Autodesk Inventor part; units mm, degrees
ref_plane "YZ Plane" through (0, 0, 0) normal (1, 0, 0) x (0, 1, 0)
ref_plane "XZ Plane" through (0, 0, 0) normal (0, 1, 0) x (-1, 0, 0)
ref_plane "XY Plane" through (0, 0, 0) normal (0, 0, 1) x (1, 0, 0)
sketch "スケッチ1" plane through (0, 0, 0) normal (0, 0, 1) x (1, 0, 0)
  line L0 (-10, 30) -> (10, 30)
  line L1 (10, 30) -> (10, -30)
  line L2 (10, -30) -> (-10, -30)
  line L3 (-10, -30) -> (-10, 30)
  line L4 (-10, 30) -> (10, -30) construction
  line L5 (10, 30) -> (-10, -30) construction
  line L6 (10, 30) -> (20, 30)
  line L7 (20, 30) -> (20, 11)
  line L8 (20, 11) -> (10, 11)
  line L9 (10.5, 30) -> (10.5, 11) construction
  circle A0 centre (10.5, 24) radius 1.25
  circle A1 centre (10.5, 16) radius 1.25
  line L10 (3.5, 30) -> (3.5, 11)
  line L11 (3.5, 11) -> (-10, 11)
  circle A2 centre (-6.25, -26.44) radius 1.1
  line L12 (-10, -26.44) -> (10, -26.44) construction
  circle A3 centre (6.25, -26.44) radius 1.1
  line L13 (0, -30) -> (0, 30) construction
  line L14 (-9.5, -15.94) -> (9.5, -15.94)
  line L15 (9.5, -15.94) -> (9.5, -18.94)
  line L16 (9.5, -18.94) -> (-9.5, -18.94)
  line L17 (-9.5, -18.94) -> (-9.5, -15.94)
  line L18 (-9.5, -15.94) -> (9.5, -18.94) construction
  line L19 (9.5, -15.94) -> (-9.5, -18.94) construction
  line L20 (10, 11) -> (3.5, 11)
  circle A4 centre (6.25, -26.44) radius 2.5
  circle A5 centre (-6.25, -26.44) radius 2.5
  line L21 (10, -30) -> (12, -30)
  line L22 (12, -30) -> (12, 11)
  line L23 (-10, 11) -> (-12, 11)
  line L24 (-12, 11) -> (-12, -30)
  line L25 (-12, -30) -> (-10, -30)
  point P0 (0, 0)
  point P1 (0, -17.44)
  dimension "d0" = 60
  dimension "d1" = 20
  dimension "d2" = 2.5
  dimension "d3" = 8
  dimension "d4" = 5
  dimension "d5" = 10.5
  dimension "d6" = 19
  dimension "d7" = 10
  dimension "d8" = 7
  dimension "d9" = 2.2
  dimension "d10" = 2.2
  dimension "d11" = 12.5
  dimension "d12" = 6.25
  dimension "d13" = 3.56
  dimension "d14" = 3
  dimension "d15" = 19
  dimension "d16" = 9
  dimension "d22" = 5
  dimension "d23" = 5
  dimension "d27" = 2
  dimension "d28" = 2
extrude "押し出し1" add sketch "スケッチ1" along normal blind 2 contours L0 L1 A0 A1 L20 L10 | L11 L20 L1 L2 L3 | L6 L7 L8 L1 A1 A0 | A4 | A5
extrude "押し出し2" add sketch "スケッチ1" against normal blind 2.95 contours L0 L1 A0 A1 L20 L10 | L6 L7 L8 L1 A1 A0
fillet "フィレット1" radius 8 2 edges at (10, 11, 1) (3.5, 11, 1)
extrude "押し出し3" cut sketch "スケッチ1" along normal blind 1 contours A4 | A5
fillet "フィレット2" radius 8 1 edges at (-10, 11, 1)
extrude "押し出し4" add sketch "スケッチ1" along normal up to surface (2 mm away) contours L11 L20 L1 L2 L3 | L3 L25 L24 L23 | L8 L22 L21 L1
properties part number "adapter_tof"
Could you check a few things on this model? Use its own coordinates, in mm. A direction names the side the tool comes from. Coordinates: 2 decimals unless noted, no trailing zeros. Order: outer loops, then holes, each group sorted by start corner. A loop starts at its lowest first (then second) coordinate and runs counter-clockwise, first axis right, second up. Notation, with made-up numbers: M 53,33.25 L 72,33.25 A13 ccw 72,58.25 Z; hole C 11.25,3.5 d1. An arc over 180 degrees is marked long. Use a Markdown table: item, result. Add a question column.
Q1. I want a section at C-C on y = -26.44. List the corners of the cut face in (x, z) for me, then the cut area to 3 significant figures.
Q2. I want a section at A-A on x = -6.25. List the corners of the cut face in (y, z) for me, then the cut area to 3 significant figures.
Q3. I'm going to push flat-ended pins straight in: pin 1 (0.6 mm diameter, centred on x = -6.5, z = 1.5, fed in from +Y); pin 2 (12 mm diameter, centred on x = 16, y = -1.5, fed in from -Z); pin 3 (0.6 mm diameter, centred on y = -18, z = 0.5, fed in from +X); pin 4 (1 mm diameter, centred on y = -6.5, z = -2, fed in from -X). Where does each tip first touch, or does it pass through?
Q4. I want a section at B-B on y = 24. List the corners of the cut face in (x, z) for me.
Q5. I want a section at D-D on x = -1.5. List the corners of the cut face in (y, z) for me, then the cut area to 3 significant figures.
Q6. We'd pull the mould along X, two halves only. Please class faces 5 (the flat face through (0, -18.94, 1)), 6 (the cylindrical face through (1.53, 13.74, 1.01)), 7 (the flat face through (12, 11, -2)): pulls with the +X half, pulls with the -X half, needs draft (parallel to the pull), parting line crosses it, or undercut.
Q7. Which directions (+Z, -Z, +X, -X, +Y, -Y) give clear straight access to the entire face, cutting with the end or side of a thin tool? Please do faces 1 (the cylindrical face through (-5.1, -24.22, 0.49)), 2 (the flat face through (0, -15.94, 1)), 3 (the flat face through (3.5, 23, -1)), 4 (the flat face through (-8, 11, 1)).
Q8. If I drill on L1, parallel to X at y = -26.5, z = 0.05; L2, parallel to Y at x = 6.25, z = 1.3; L3, parallel to Y at x = 10.5, z = -0.3, over which ranges is the centre line in solid material (lowest first)?
Checked values:
| question | item | result |
|---|---|---|
| 1 | outline | M -12,0 L -8.75,0 L -8.75,1 L -7.35,1 L -7.35,2 L -12,2 Z; M -5.15,1 L -3.75,1 L -3.75,0 L 3.75,0 L 3.75,1 L 5.15,1 L 5.15,2 L -5.15,2 Z; M 7.35,1 L 8.75,1 L 8.75,0 L 12,0 L 12,2 L 7.35,2 Z |
| 1 | area | 33.6 mm² |
| 2 | outline | M -30,0 L -28.94,0 L -28.94,1 L -27.54,1 L -27.54,2 L -30,2 Z; M -25.34,1 L -23.94,1 L -23.94,0 L -18.94,0 L -18.94,2 L -25.34,2 Z; M -15.94,0 L 11,0 L 11,2 L -15.94,2 Z |
| 2 | area | 68.8 mm² |
| 3 | pin 1 | y = 11 |
| 3 | pin 2 | z = 0 |
| 3 | pin 3 | x = 12 |
| 3 | pin 4 | through |
| 4 | outline | M 3.5,-2.95 L 9.25,-2.95 L 9.25,2 L 3.5,2 Z; M 11.75,-2.95 L 20,-2.95 L 20,2 L 11.75,2 Z |
| 5 | outline | M -30,0 L -18.94,0 L -18.94,2 L -30,2 Z; M -15.94,0 L 11.58,0 L 11.58,2 L -15.94,2 Z |
| 5 | area | 77.2 mm² |
| 6 | face 5 | undercut |
| 6 | face 6 | pulls with the -X half |
| 6 | face 7 | needs draft |
| 7 | face 1 | -Z |
| 7 | face 2 | +Z, -Z |
| 7 | face 3 | -Z, -X, +Y |
| 7 | face 4 | +Z, -Z, -X, +Y |
| 8 | L1 | -12 to -8.75, -3.75 to 3.75, 8.75 to 12 |
| 8 | L2 | -30 to -27.54, -25.34 to -18.94, -15.94 to 30 |
| 8 | L3 | 11 to 14.75, 17.25 to 22.75, 25.25 to 30 |
